Design review of the part built by this model. Coordinates are the model's own, in mm. Round coordinates to 2 decimals unless told otherwise and drop trailing zeros. Write item = value, one per line.
from build123d import *

# Parameters (mm, degrees)
SKETCH1_W            = 1094.236516538
SKETCH1_H            = 400
BOSS_EXTRUDE1_DEPTH  = 18
CAVITY1_START        = -33
CAVITY1_OUTLINE_W    = 18
CAVITY1_OUTLINE_H    = 18
CAVITY1_DEPTH        = 30
CAVITY1_START_2      = 399.118258269
CAVITY1_2_OUTLINE_W  = 18
CAVITY1_2_OUTLINE_H  = 18
CAVITY1_2_DEPTH      = 30
CAVITY1_START_3      = 813.236516538
CAVITY1_3_OUTLINE_W  = 18
CAVITY1_3_OUTLINE_H  = 18
CAVITY1_3_DEPTH      = 30
CAVITY1_START_4      = -15
CAVITY1_4_OUTLINE_W  = 18
CAVITY1_4_OUTLINE_H  = 18
CAVITY1_4_DEPTH      = 50
CAVITY1_START_5      = 831.236516538
CAVITY1_5_OUTLINE_W  = 18
CAVITY1_5_OUTLINE_H  = 18
CAVITY1_5_DEPTH      = 30
CAVITY1_START_6      = 169.118258269
CAVITY1_6_OUTLINE_W  = 18
CAVITY1_6_OUTLINE_H  = 18
CAVITY1_6_DEPTH      = 30
CAVITY1_START_7      = 629.118258269
CAVITY1_7_OUTLINE_W  = 18
CAVITY1_7_OUTLINE_H  = 18
CAVITY1_7_DEPTH      = 30
CAVITY1_START_8      = -35
CAVITY1_8_OUTLINE_W  = 18
CAVITY1_8_OUTLINE_H  = 18
CAVITY1_8_DEPTH      = 50
CAVITY1_START_9      = 389.118258269
CAVITY1_9_OUTLINE_W  = 18
CAVITY1_9_OUTLINE_H  = 18
CAVITY1_9_DEPTH      = 50
CAVITY1_START_10     = 793.236516538
CAVITY1_10_OUTLINE_W = 18
CAVITY1_10_OUTLINE_H = 18
CAVITY1_10_DEPTH     = 20
CAVITY1_START_11     = 861.236516538
CAVITY1_11_OUTLINE_W = 18
CAVITY1_11_OUTLINE_H = 18
CAVITY1_11_DEPTH     = 2
SKETCH2_W            = 18
SKETCH2_H            = 50
CUT_EXTRUDE1_DEPTH   = 18
M3_CLEARANCE_HOLE1_D = 3.4
SKETCH5_R            = 3
CUT_EXTRUDE2_DEPTH   = 30


# Read off the part's stored shape, not the designer's step: Cavity1
with BuildPart() as part:
    # Sketch1 → Boss-Extrude1 (new body)
    with BuildSketch(Plane.XY):
        with Locations((414.118258269, 20)):
            Rectangle(SKETCH1_W, SKETCH1_H)
    extrude(amount=BOSS_EXTRUDE1_DEPTH)

    # Cavity1 outline → Cavity1 (cut)
    with BuildSketch(Plane.YZ.offset(CAVITY1_START)):
        with Locations((-9, 9)):
            Rectangle(CAVITY1_OUTLINE_W, CAVITY1_OUTLINE_H)
        with Locations((39.65, 9)):
            Rectangle(CAVITY1_OUTLINE_W, CAVITY1_OUTLINE_H)
    extrude(amount=CAVITY1_DEPTH, mode=Mode.SUBTRACT)

    # Cavity1 2 outline → Cavity1 2 (cut)
    with BuildSketch(Plane.YZ.offset(CAVITY1_START_2)):
        with Locations((-171, 9)):
            Rectangle(CAVITY1_2_OUTLINE_W, CAVITY1_2_OUTLINE_H)
        with Locations((39.65, 9)):
            Rectangle(CAVITY1_2_OUTLINE_W, CAVITY1_2_OUTLINE_H)
    extrude(amount=CAVITY1_2_DEPTH, mode=Mode.SUBTRACT)

    # Cavity1 3 outline → Cavity1 3 (cut)
    with BuildSketch(Plane.YZ.offset(CAVITY1_START_3)):
        with Locations((-9, 9)):
            Rectangle(CAVITY1_3_OUTLINE_W, CAVITY1_3_OUTLINE_H)
        with Locations((-171, 9)):
            Rectangle(CAVITY1_3_OUTLINE_W, CAVITY1_3_OUTLINE_H)
    extrude(amount=CAVITY1_3_DEPTH, mode=Mode.SUBTRACT)

    # Cavity1 4 outline → Cavity1 4 (cut)
    with BuildSketch(Plane.YZ.offset(CAVITY1_START_4)):
        with Locations((-171, 9)):
            Rectangle(CAVITY1_4_OUTLINE_W, CAVITY1_4_OUTLINE_H)
    extrude(amount=CAVITY1_4_DEPTH, mode=Mode.SUBTRACT)

    # Cavity1 5 outline → Cavity1 5 (cut)
    with BuildSketch(Plane.YZ.offset(CAVITY1_START_5)):
        with Locations((-9, 9)):
            Rectangle(CAVITY1_5_OUTLINE_W, CAVITY1_5_OUTLINE_H)
        with Locations((39.65, 9)):
            Rectangle(CAVITY1_5_OUTLINE_W, CAVITY1_5_OUTLINE_H)
    extrude(amount=CAVITY1_5_DEPTH, mode=Mode.SUBTRACT)

    # Cavity1 6 outline → Cavity1 6 (cut)
    with BuildSketch(Plane.YZ.offset(CAVITY1_START_6)):
        with Locations((39.65, 9)):
            Rectangle(CAVITY1_6_OUTLINE_W, CAVITY1_6_OUTLINE_H)
    extrude(amount=CAVITY1_6_DEPTH, mode=Mode.SUBTRACT)

    # Cavity1 7 outline → Cavity1 7 (cut)
    with BuildSketch(Plane.YZ.offset(CAVITY1_START_7)):
        with Locations((39.65, 9)):
            Rectangle(CAVITY1_7_OUTLINE_W, CAVITY1_7_OUTLINE_H)
    extrude(amount=CAVITY1_7_DEPTH, mode=Mode.SUBTRACT)

    # Cavity1 8 outline → Cavity1 8 (cut)
    with BuildSketch(Plane.YZ.offset(CAVITY1_START_8)):
        with Locations((-9, 9)):
            Rectangle(CAVITY1_8_OUTLINE_W, CAVITY1_8_OUTLINE_H)
    extrude(amount=CAVITY1_8_DEPTH, mode=Mode.SUBTRACT)

    # Cavity1 9 outline → Cavity1 9 (cut)
    with BuildSketch(Plane.YZ.offset(CAVITY1_START_9)):
        with Locations((-171, 9)):
            Rectangle(CAVITY1_9_OUTLINE_W, CAVITY1_9_OUTLINE_H)
    extrude(amount=CAVITY1_9_DEPTH, mode=Mode.SUBTRACT)

    # Cavity1 10 outline → Cavity1 10 (cut)
    with BuildSketch(Plane.YZ.offset(CAVITY1_START_10)):
        with Locations((-171, 9)):
            Rectangle(CAVITY1_10_OUTLINE_W, CAVITY1_10_OUTLINE_H)
    extrude(amount=CAVITY1_10_DEPTH, mode=Mode.SUBTRACT)

    # Cavity1 11 outline → Cavity1 11 (cut)
    with BuildSketch(Plane.YZ.offset(CAVITY1_START_11)):
        with Locations((-9, 9)):
            Rectangle(CAVITY1_11_OUTLINE_W, CAVITY1_11_OUTLINE_H)
    extrude(amount=CAVITY1_11_DEPTH, mode=Mode.SUBTRACT)

    # Sketch2 → Cut-Extrude1 (cut)
    with BuildSketch(Plane.XY.offset(18)):
        with Locations((952.236516538, 145)):
            Rectangle(SKETCH2_W, SKETCH2_H)
        with Locations((952.236516538, -105)):
            Rectangle(SKETCH2_W, SKETCH2_H)
        with Locations((-124, -105)):
            Rectangle(SKETCH2_W, SKETCH2_H)
        with Locations((-124, 145)):
            Rectangle(SKETCH2_W, SKETCH2_H)
    extrude(amount=-CUT_EXTRUDE1_DEPTH, mode=Mode.SUBTRACT)

    # M3 Clearance Hole1 (through all)
    with Locations(Plane.XY.offset(18)):
        with Locations((-65, -171), (212.059129134, -171), (616.177387403, -171), (903.236516538, -171), (952.236516538, -155), (903.236516538, -9), (952.236516538, 20), (902.236516538, 39.65), (952.236516538, 195), (-124, 195), (-124, 20), (-124, -155), (-75, -9), (-74, 39.65), (299.118258269, 39.65), (529.118258269, 39.65)):
            Hole(M3_CLEARANCE_HOLE1_D / 2)

    # Sketch5 → Cut-Extrude2 (cut)
    with BuildSketch(Plane.XY.offset(18)):
        with Locations((-117.121320344, 167.878679656)):
            Circle(SKETCH5_R)
        with Locations((-117.121320344, 122.121320344)):
            Circle(SKETCH5_R)
        with Locations((-30.878679656, 46.528679656)):
            Circle(SKETCH5_R)
        with Locations((-30.878679656, 32.771320344)):
            Circle(SKETCH5_R)
        with Locations((-5.121320344, 32.771320344)):
            Circle(SKETCH5_R)
        with Locations((-5.121320344, 46.528679656)):
            Circle(SKETCH5_R)
        with Locations((-32.878679656, -2.121320344)):
            Circle(SKETCH5_R)
        with Locations((-32.878679656, -15.878679656)):
            Circle(SKETCH5_R)
        with Locations((12.878679656, -15.878679656)):
            Circle(SKETCH5_R)
        with Locations((12.878679656, -2.121320344)):
            Circle(SKETCH5_R)
        with Locations((-117.121320344, -82.121320344)):
            Circle(SKETCH5_R)
        with Locations((-117.121320344, -127.878679656)):
            Circle(SKETCH5_R)
        with Locations((945.357836881, -127.878679656)):
            Circle(SKETCH5_R)
        with Locations((945.357836881, -82.121320344)):
            Circle(SKETCH5_R)
        with Locations((945.357836881, 122.121320344)):
            Circle(SKETCH5_R)
        with Locations((945.357836881, 167.878679656)):
            Circle(SKETCH5_R)
        with Locations((815.357836881, -2.121320344)):
            Circle(SKETCH5_R)
        with Locations((815.357836881, -15.878679656)):
            Circle(SKETCH5_R)
        with Locations((861.115196194, -15.878679656)):
            Circle(SKETCH5_R)
        with Locations((861.115196194, -2.121320344)):
            Circle(SKETCH5_R)
        with Locations((171.241320344, 46.528679656)):
            Circle(SKETCH5_R)
        with Locations((171.241320344, 32.771320344)):
            Circle(SKETCH5_R)
        with Locations((196.998679656, 32.771320344)):
            Circle(SKETCH5_R)
        with Locations((196.998679656, 46.528679656)):
            Circle(SKETCH5_R)
        with Locations((631.237836881, 46.528679656)):
            Circle(SKETCH5_R)
        with Locations((631.237836881, 32.771320344)):
            Circle(SKETCH5_R)
        with Locations((656.995196194, 32.771320344)):
            Circle(SKETCH5_R)
        with Locations((656.995196194, 46.528679656)):
            Circle(SKETCH5_R)
        with Locations((833.357836881, 46.528679656)):
            Circle(SKETCH5_R)
        with Locations((833.357836881, 32.771320344)):
            Circle(SKETCH5_R)
        with Locations((859.115196194, 32.771320344)):
            Circle(SKETCH5_R)
        with Locations((859.115196194, 46.528679656)):
            Circle(SKETCH5_R)
        with Locations((401.241320344, 46.528679656)):
            Circle(SKETCH5_R)
        with Locations((401.241320344, 32.771320344)):
            Circle(SKETCH5_R)
        with Locations((426.998679656, 32.771320344)):
            Circle(SKETCH5_R)
        with Locations((426.998679656, 46.528679656)):
            Circle(SKETCH5_R)
        with Locations((-15, -162)):
            Circle(SKETCH5_R)
        with Locations((35, -162)):
            Circle(SKETCH5_R)
        with Locations((793.236516538, -162)):
            Circle(SKETCH5_R)
        with Locations((843.236516538, -162)):
            Circle(SKETCH5_R)
        with Locations((389.12, -162)):
            Circle(SKETCH5_R)
        with Locations((439.12, -162)):
            Circle(SKETCH5_R)
    extrude(amount=-CUT_EXTRUDE2_DEPTH, mode=Mode.SUBTRACT)


solid = part.part
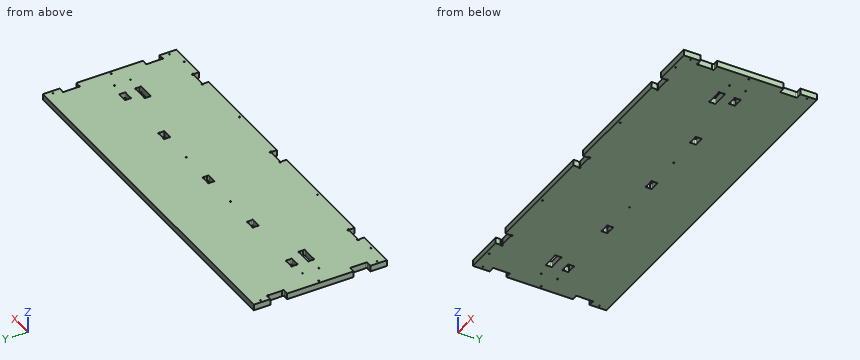
1) We need section A-A on z = 5.5. Give the number of separate pieces and of enclosed holes in the cut face, and give its area (3 significant figures).
Findings:
separate_pieces = 1
enclosed_holes = 23
area = 426,000 mm^2
2) Clearance check with a flat-ended pin moving along its axis: pin 1 Ø3 at (y, z) = (-108.5, 3) entering from -X. State where the tip first meets the part, or that it passes through.
Findings:
pin_1 = -115
3) To check wall thickness, follow L1, parallel to Y at x = 13, z = 9; L2, parallel to Y at x = 189, z = 1.75; L3, parallel to X at y = 127, z = 2. State the ranges of each line that lie inside material, in increasing order. Write a range as from..to.
Findings:
L1 = -162..-18.88, 0.88..220
L2 = -180..30.65, 48.65..220
L3 = -115..943.24
